Part model, mm, in its own coordinate system. Face numbers are marked on the shaded views. A direction names the side the tool comes from. Round coordinates to 2 decimals unless told otherwise and drop trailing zeros. Write each loop counter-clockwise with the first axis right and the second up, starting at its lowest first coordinate (ties: lowest second). Pieces come first, ordered by that corner, then holes. Notation, with made-up numbers: M -38.75,-4.5 L -10.75,-4.5 A30 cw -10.75,25.5 Z; hole C 30,14.25 d7. An arc over 180 degrees is marked long. Use a Markdown table: item, result. Add a question column.
1) Slice it at B-B on x = 0. Write the cut outline in (y, z).
2) Slice it at C-C on x = 4. Write the cut outline in (y, z).
3) Slice it at D-D on y = 10.25. Write the cut outline in (x, z), plus the area to 3 significant figures.
4) Two-plate mould, pull along Y, no slides. Class the marked faces 1, 2, 3 and 4: released by +Y, released by -Y, zero draft, split by the parting line, or undercut.
5) Drop flat-ended pins along their axis: P1, Ø2, axis at x = 1, y = 9.5, coming from the +Z side; P2, Ø2, axis at x = -4, y = 2.5, coming from the -Z side; P3, Ø2, axis at x = 5, z = -13, coming from the -Y side; P4, Ø4, axis at x = -5.5, y = 5.5, coming from the +Z side. Give the stop position or say it passes through.
6) Slice it at A-A on y = 1.75. Write the cut outline in (x, z).
7) Which spindle directions (+Z, -Z, +X, -X, +Y, -Y) get a long thin tool onto all of the face, cutting with end or side? Do the marked faces 5, 6 and 7. Say none if no direction does.
8) Wall check: probe 1 along X at (y, z) = (1.5, -8.25); probe 2 along Y at (x, z) = (1.5, -10.25); probe 3 along Z at (x, y) = (0, 0.3). Give the ranges that are in metal, low to high.
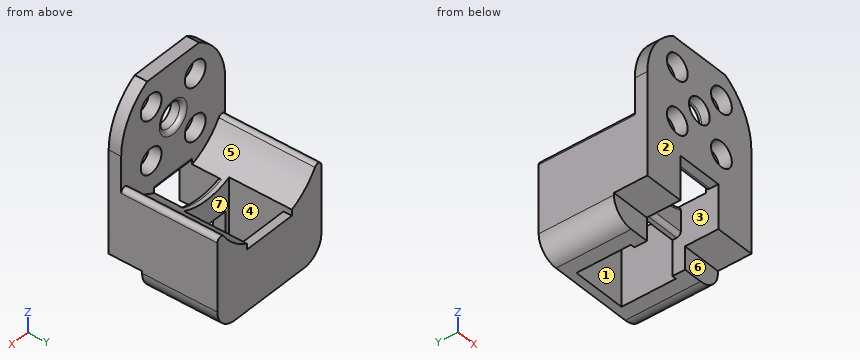
Autodesk Inventor part; units mm, degrees
ref_plane "Pracovní rovina1" through (0, 1.5, 0) normal (0, 1, 0) x (1, 0, 0)
ref_plane "Pracovní rovina2" through (-2.75, 0, -15) normal (0, 0, -1) x (-1, 0, 0)
ref_plane "Pracovní rovina3" through (0, 13, 0) normal (0, 1, 0) x (1, 0, 0)
sketch "Náčrt1" plane through (0, 0, 0) normal (0, 1, 0) x (-1, 0, 0)
  arc A0 (2.75, -6.9776) -> (-2.75, -6.9776) centre (0, 0) ccw
  line L0 (-7.5, 0) -> (-7.5, -15)
  line L1 (7.5, -15) -> (7.5, 0)
  line L2 (2.75, -6.9776) -> (-2.75, -6.9776)
  line L3 (-2.75, -6.9776) -> (-2.75, -15)
  line L4 (2.75, -15) -> (2.75, -6.9776)
  circle A1 centre (4.5, 0) radius 1.5
  circle A2 centre (0, 0) radius 1.5
  circle A3 centre (0, 4.5) radius 1.5
  circle A4 centre (-4.5, 0) radius 1.5
  circle A5 centre (0, -4.5) radius 1.5
  line L5 (-7.5, -15) -> (-2.75, -15)
  line L6 (2.75, -15) -> (7.5, -15)
  circle A6 centre (3.182, 3.182) radius 1.5
  circle A7 centre (0, 4.5) radius 1.5
  circle A8 centre (-3.182, 3.182) radius 1.5
  circle A9 centre (-4.5, 0) radius 1.5
  circle A10 centre (-3.182, -3.182) radius 1.5
  circle A11 centre (0, -4.5) radius 1.5
  circle A12 centre (3.182, -3.182) radius 1.5
  line L7 (-1.5, 0) -> (-3, 0)
  line L8 (-6, 0) -> (-7.5, 0)
  line L9 (7.5, 0) -> (6, 0)
  line L10 (3, 0) -> (1.5, 0)
  dimension "d0" = 15
  dimension "d1" = 3
  dimension "d2" = 3
  dimension "d5" = 360
  dimension "d7" = 4.5
  dimension "d8" = 5.5
  dimension "d9" = 15
  dimension "d10" = 15
  dimension "d13" = 360
extrude "Vysunutí1" add sketch "Náčrt1" along normal blind 1.5 contours L2 A0 L8 A4 L7 A2 L10 A1 L9 | A0 L1 L6 L4 | L9 A1 L10 A2 L7 A4 L8 A0 | L3 L5 L0 A0 | A1 | A4 | A3 | A5
ref_plane "Pracovní rovina1" through (0, 1.5, 0) normal (0, 1, 0) x (1, 0, 0)
sketch "Náčrt3" plane through (0, 1.5, 0) normal (0, 1, 0) x (1, 0, 0)
  arc A0 (7.5, 1.9526) -> (-7.5, 1.9526) centre (0, 0) ccw
  line L0 (-7.5, 15) -> (-7.5, 0)
  line L1 (7.5, 15) -> (2.75, 15)
  line L2 (7.5, 1.9526) -> (7.5, 15)
  line L3 (7.5, 15) -> (-7.5, 15)
  line L4 (-7.5, 15) -> (-7.5, 1.9526)
  dimension "d18" = 15.5
extrude "Vysunutí2" add sketch "Náčrt3" along normal blind 11.5
ref_plane "Pracovní rovina2" through (-2.75, 0, -15) normal (0, 0, -1) x (-1, 0, 0)
sketch "Náčrt4" plane through (-2.75, 0, -15) normal (0, 0, -1) x (-1, 0, 0)
  line L0 (-5.5, 0) -> (-5.5, 1.5)
  line L1 (-5.5, 1.5) -> (0, 1.5)
  line L2 (0, 1.5) -> (0, 4.5)
  line L3 (0, 4.5) -> (-5.5, 4.5)
  line L4 (-5.5, 4.5) -> (-5.5, 1.5)
  point P0 (-2.75, 0)
  dimension "d51" = 3
extrude "Vysunutí3" cut sketch "Náčrt4" against normal blind 9
fillet "Zaoblení1" radius 0.5 1 edges at (7.5, 7.25, -1.9526)
fillet "Zaoblení2" radius 0.5 1 edges at (-7.5, 7.25, -1.9526)
sketch "Náčrt9" plane through (-2.75, 0, -15) normal (0, 0, -1) x (-1, 0, 0)
  line L0 (0, 0) -> (0, 4.5)
  line L1 (0, 0) -> (4.75, 0)
  line L2 (4.75, 0) -> (4.75, 13)
  line L3 (-10.25, 13) -> (4.75, 13)
  line L4 (-10.25, 0) -> (-10.25, 13)
  line L5 (-10.25, 0) -> (-5.5, 0)
  line L6 (-5.5, 0) -> (-5.5, 4.5)
  line L7 (-6, 5.5) -> (0.5, 5.5)
  line L8 (0.5, 5.5) -> (0.5, 12)
  line L9 (0.5, 12) -> (-6, 12)
  line L10 (-6, 12) -> (-6, 5.5)
  line L11 (-5.5, 4.5) -> (0, 4.5)
  point P0 (-2.75, 0)
  dimension "d28" = 6.5
  dimension "d29" = 6.5
  dimension "d31" = 0.5
  dimension "d50" = 1
extrude "Vysunutí5" cut sketch "Náčrt9" against normal blind 8 contours L10 L9 L8 L7
fillet "Zaoblení4" radius 0.5 1 edges at (1.5, 1.5, 0)
fillet "Zaoblení5" radius 2.5 2 edges at (-7.5, 6.5, -15) (7.5, 6.5, -15)
fillet "Zaoblení6" radius 0.5 2 edges at (0, 4.5, -7.75) (0, 1.5, -6.9776)
ref_plane "Pracovní rovina3" through (0, 13, 0) normal (0, 1, 0) x (1, 0, 0)
sketch "Náčrt10" plane through (0, 13, 0) normal (0, 1, 0) x (1, 0, 0)
  arc A0 (3.25, 7.0356) -> (-3.25, 7.0356) centre (0, 0) ccw
  line L0 (-3.25, 15) -> (-3.25, 7.0356)
  line L1 (3.25, 15) -> (-3.25, 15)
  line L2 (3.25, 15) -> (3.25, 7.0356)
  line L3 (3.25, 7.0356) -> (-3.25, 7.0356)
  line L4 (-3.25, 7.0356) -> (-3.25, 7.75)
  line L5 (-3.25, 7.75) -> (3.25, 7.75)
  line L6 (3.25, 7.75) -> (3.25, 7.0356)
extrude "Vysunutí6" cut sketch "Náčrt10" against normal blind 2 contours L3 A0 | A0 L5 L2 | A0 L0 L5
sketch "Sketch11" plane through (-7.5, 0, 0) normal (-1, 0, 0) x (0, 0, 1)
  line L0 (-15, 0) -> (-6.9776, 0)
  line L1 (-15, 0) -> (-12.25, 0)
  line L2 (-12.25, 0) -> (-12.25, 4)
  line L3 (-12.25, 4) -> (-15, 4)
  line L4 (-15, 4) -> (-15, 0)
  point P0 (0, 0)
  dimension "d42" = 2.75
  dimension "d43" = 4
extrude "Extrusion7" cut sketch "Sketch11" against normal through all
sketch "Sketch12" plane through (0, 0, 0) normal (0, -1, 0) x (1, 0, 0)
  line L0 (7.5804, 6.5) -> (-7.5515, 6.5)
  line L1 (-7.5515, 6.5) -> (-7.5515, 9.7793)
  line L2 (-7.5515, 9.7793) -> (7.5804, 9.7793)
  line L3 (7.5804, 9.7793) -> (7.5804, 6.5)
  arc A0 (7.5, 0) -> (-7.5, 0) centre (0, 0) ccw
  dimension "d46" = 1
extrude "Extrusion8" cut sketch "Sketch12" against normal through all
sketch "Sketch13" plane through (-2.75, 1.5, -7.2457) normal (1, 0, 0) x (0, 0, -1)
  line L0 (7.7543, 2.5) -> (7.7543, 3)
  line L1 (7.7543, 3) -> (3.5043, 3)
  line L2 (3.5043, 3) -> (3.5043, 4)
  line L3 (3.5043, 4) -> (7.7543, 4)
  line L4 (7.7543, 4) -> (7.7543, 3)
  line L5 (5.0043, -1.5) -> (5.0043, 2.5)
  point P0 (-7.2457, -1.5)
  dimension "d52" = 1.5
extrude "Extrusion9" cut sketch "Sketch13" along normal up to surface (5.5 mm away)
fillet "Fillet8" radius 0.5 1 edges at (0, 4.5, -10.75)
equation "\"d9\" = d0"
equation "\"d29\" = d28"
equation "\"d31\" = -0.5 * d8 + 0.5 * d28"
properties part number "uchyt motoru-final"
Entries:
| question | item | result |
|---|---|---|
| 1 | outline | M 0,-6.98 L 1,-6.98 A0.5 ccw 1.5,-6.48 L 1.5,-2 A0.5 ccw 1,-1.5 L 0,-1.5 Z; M 0,1.5 L 1,1.5 A0.5 ccw 1.5,2 L 1.5,6.5 L 0,6.5 Z; M 4.5,-10.25 A0.5 ccw 5,-10.75 L 5.5,-10.75 L 5.5,-7.75 L 5,-7.75 A0.5 ccw 4.5,-8.25 Z; M 12,-15 L 13,-15 L 13,-7.75 L 12,-7.75 Z |
| 2 | outline | M 0,-12.25 L 4,-12.25 L 4,-15 L 13,-15 L 13,-6.64 L 1.5,-6.64 L 1.5,-4.44 L 0,-4.44 Z; M 0,-1.92 L 1.5,-1.92 L 1.5,1.92 L 0,1.92 Z; M 0,4.44 L 1.5,4.44 L 1.5,6.34 L 0,6.34 Z |
| 3 | outline | M -7.5,-12.5 A2.5 ccw -5,-15 L -3.25,-15 L -3.25,-7.04 A7.75 cw -6.58,-4.1 A0.5 ccw -7.5,-4.37 Z; M 3.25,-15 L 5,-15 A2.5 ccw 7.5,-12.5 L 7.5,-4.37 A0.5 ccw 6.58,-4.1 A7.75 cw 3.25,-7.04 Z |
| 3 | area | 78.5 mm^2 |
| 4 | face 1 | undercut |
| 4 | face 2 | released by -Y |
| 4 | face 3 | zero draft |
| 4 | face 4 | undercut |
| 5 | P1 | passes through |
| 5 | P2 | stops at z = -12.25 |
| 5 | P3 | stops at y = 0 |
| 5 | P4 | stops at z = -3.87 |
| 6 | outline | M -7.5,-12.25 L -2.75,-12.25 L -2.75,-7.25 A7.75 cw -6.58,-4.1 A0.5 ccw -7.5,-4.37 Z; M 2.75,-12.25 L 7.5,-12.25 L 7.5,-4.37 A0.5 ccw 6.58,-4.1 A7.75 cw 2.75,-7.25 Z |
| 7 | face 5 | +Z, +Y |
| 7 | face 6 | -Z, +X, -X, -Y |
| 7 | face 7 | +Z, -Z |
| 8 | probe 1 | x = -7.5 to -2.75, 2.75 to 7.5 |
| 8 | probe 2 | y = 4.5 to 5.5, 12 to 13 |
| 8 | probe 3 | z = -6.98 to -1.5, 1.5 to 6.5 |
